Geometry: final body of the model. Coordinates: model frame, mm. Face numbers are marked on the shaded views. A direction names the side the tool comes from. Give positions to 0.01 mm unless a question says otherwise; leave off trailing zeros. Write each loop counter-clockwise with the first axis right and the second up, starting at its lowest first coordinate (ties: lowest second). Pieces come first, ordered by that corner, then holes. Notation, with made-up numbers: M 3,35.25 L 62,35.25 A26 cw 62,57.25 Z; hole C -10.5,-38.75 d8. An arc over 180 degrees is marked long. Use a Markdown table: item, result. Add a question column.
(1) Cut plane B-B (y = 0). Output: boundary loops of the cut face in (x, z).
(2) Draft query along Y for the marked faces 1, 2 and 3. Return one class per face: released by +Y, released by -Y, zero draft, split by the parting line, or undercut.
(3) Pin query (flat end, axial travel): pin 1 Ø3 at (x, z) = (-2.5, 8.5) entering from +Y; pin 2 Ø3 at (x, y) = (6.5, 0.5) entering from +Z; pin 3 Ø3 at (x, z) = (7, 2) entering from +Y. Return the tip coordinate at first contact, or that it passes through.
(4) Material intervals for L1, parallel to Z at x = -7.5, y = -0.25; L2, parallel to Y at x = -1, z = 4.25; L3, parallel to Y at x = 0.5, z = 8.75, sorted ascending.
(5) Reachability of the marked faces 4, 5, 6, 7 and 8 from +Z, -Z, +X, -X, +Y, -Y: full face, straight path, thin tool, end or side. Return the list, or none.
(6) Cut plane A-A (x = 0). Output: boundary loops of the cut face in (y, z).
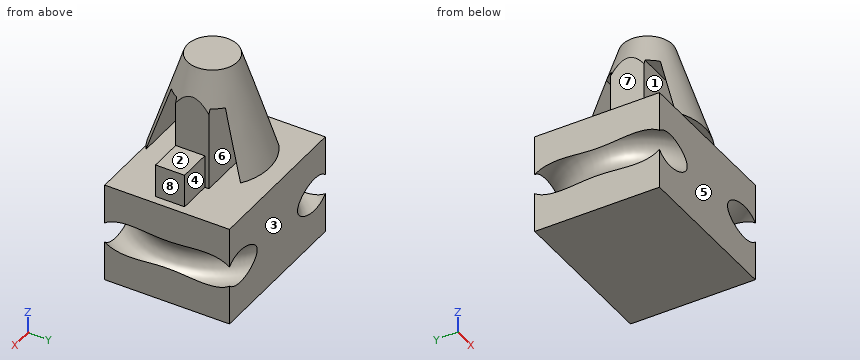
```python
from build123d import *

# Parameters (mm, degrees)
BOX008_W               = 10
BOX008_H               = 10
BOX008_DEPTH           = 5
BOX009_W               = 10
BOX009_H               = 10
BOX009_DEPTH           = 5
BOX006_W               = 10
BOX006_H               = 10
BOX006_DEPTH           = 15
BOX006_PLACEMENT_ANGLE = 90
BOX005_W               = 10
BOX005_H               = 10
BOX005_DEPTH           = 15
BOX002_W               = 20
BOX002_H               = 8
BOX002_DEPTH           = 18
BOX002_ROLL_ANGLE      = 16.999951
BOX003_W               = 20
BOX003_H               = 5
BOX003_DEPTH           = 10
CUT001_PLACEMENT_ANGLE = 180
BOX001_W               = 20
BOX001_H               = 8
BOX001_DEPTH           = 18
BOX001_ROLL_ANGLE      = 16.999951
BOX_W                  = 20
BOX_H                  = 5
BOX_DEPTH              = 10
TORUS_R                = 2
BOX007_W               = 19
BOX007_H               = 15
BOX007_DEPTH           = 12
BOX004_W               = 11
BOX004_H               = 3.5
BOX004_DEPTH           = 4


with BuildPart() as box008:
    # Box008 → Box008 (new body)
    with BuildSketch(Plane(origin=(-5, 5, -3), x_dir=(1, 0, 0), z_dir=(0, 0, 1))):
        with Locations((5, 5)):
            Rectangle(BOX008_W, BOX008_H)
    extrude(amount=BOX008_DEPTH)


with BuildPart() as box009:
    # Box009 → Box009 (new body)
    with BuildSketch(Plane(origin=(5, -4, -3), x_dir=(-1, 0, 0), z_dir=(0, 0, 1))):
        with Locations((5, 5)):
            Rectangle(BOX009_W, BOX009_H)
    extrude(amount=BOX009_DEPTH)


with BuildPart() as box006:
    # Box006 → Box006 (new body)
    with BuildSketch(Plane.XY):
        with Locations((5, 5)):
            Rectangle(BOX006_W, BOX006_H)
    extrude(amount=BOX006_DEPTH)


with BuildPart() as box006_1:
    # Box006 placement: moved
    add(box006.part.moved(Location((-4, -4, 0))).rotate(Axis((-4, -4, 0), (0, 0, 1)), BOX006_PLACEMENT_ANGLE))


with BuildPart() as box005:
    # Box005 → Box005 (new body)
    with BuildSketch(Plane(origin=(4, -4, 0), x_dir=(1, 0, 0), z_dir=(0, 0, 1))):
        with Locations((5, 5)):
            Rectangle(BOX005_W, BOX005_H)
    extrude(amount=BOX005_DEPTH)


with BuildPart() as box002:
    # Box002 → Box002 (new body)
    with BuildSketch(Plane.XY):
        with Locations((10, 4)):
            Rectangle(BOX002_W, BOX002_H)
    extrude(amount=BOX002_DEPTH)


with BuildPart() as box002_1:
    # Box002 roll: moved
    add(box002.part.rotate(Axis((0, 0, 0), (1, 0, 0)), BOX002_ROLL_ANGLE))


with BuildPart() as box002_2:
    # Box002 placement: moved
    add(box002_1.part.moved(Location((0, 17.17, -2.83))))


with BuildPart() as cu_a001:
    # Box003 → Box003 (new body)
    with BuildSketch(Plane(origin=(0, 12, 0), x_dir=(1, 0, 0), z_dir=(0, 0, 1))):
        with Locations((10, 2.5)):
            Rectangle(BOX003_W, BOX003_H)
    extrude(amount=BOX003_DEPTH)

    # Cut001: cut Box002
    add(box002_2.part, mode=Mode.SUBTRACT)


with BuildPart() as cu_a001_1:
    # Cut001 placement: moved
    add(cu_a001.part.moved(Location((10, 10, 0))).rotate(Axis((10, 10, 0), (0, 0, 1)), CUT001_PLACEMENT_ANGLE))


with BuildPart() as box001:
    # Box001 → Box001 (new body)
    with BuildSketch(Plane.XY):
        with Locations((10, 4)):
            Rectangle(BOX001_W, BOX001_H)
    extrude(amount=BOX001_DEPTH)


with BuildPart() as box001_1:
    # Box001 roll: moved
    add(box001.part.rotate(Axis((0, 0, 0), (1, 0, 0)), BOX001_ROLL_ANGLE))


with BuildPart() as box001_2:
    # Box001 placement: moved
    add(box001_1.part.moved(Location((0, 17.17, -2.83))))


with BuildPart() as cu_a:
    # Box → Box (new body)
    with BuildSketch(Plane(origin=(0, 12, 0), x_dir=(1, 0, 0), z_dir=(0, 0, 1))):
        with Locations((10, 2.5)):
            Rectangle(BOX_W, BOX_H)
    extrude(amount=BOX_DEPTH)

    # Cut: cut Box001
    add(box001_2.part, mode=Mode.SUBTRACT)


with BuildPart() as cu_a_1:
    # Cut placement: moved
    add(cu_a.part.moved(Location((-10, -10, 0))))


with BuildPart() as cut007:
    # Cone → Cone (revolve)
    with BuildSketch(Plane.XZ):
        Polygon((0, 0), (7.5, 0), (3, 14), (0, 14), align=None)
    revolve(axis=Axis((0, 0, 0), (0, 0, 1)))

    add(cu_a_1.part, mode=Mode.SUBTRACT)

    add(cu_a001_1.part, mode=Mode.SUBTRACT)

    # Cut004: cut Box005
    add(box005.part, mode=Mode.SUBTRACT)

    # Cut005: cut Box006
    add(box006_1.part, mode=Mode.SUBTRACT)

    # Cut006: cut Box009
    add(box009.part, mode=Mode.SUBTRACT)

    # Cut007: cut Box008
    add(box008.part, mode=Mode.SUBTRACT)


with BuildPart() as torus:
    # Torus → Torus (revolve)
    with BuildSketch(Plane(origin=(-0.5, 0, -6), x_dir=(1, 0, 0), z_dir=(0, -1, 0))):
        with Locations((10.5, 0)):
            Circle(TORUS_R)
    revolve(axis=Axis((-0.5, 0, -6), (0, 0, 1)))


with BuildPart() as cut008:
    # Box007 → Box007 (new body)
    with BuildSketch(Plane(origin=(-10, -7.5, -12), x_dir=(1, 0, 0), z_dir=(0, 0, 1))):
        with Locations((9.5, 7.5)):
            Rectangle(BOX007_W, BOX007_H)
    extrude(amount=BOX007_DEPTH)

    # Cut008: cut Torus
    add(torus.part, mode=Mode.SUBTRACT)


with BuildPart() as fusion:
    # Box004 → Box004 (new body)
    with BuildSketch(Plane(origin=(-3, -2, 0), x_dir=(1, 0, 0), z_dir=(0, 0, 1))):
        with Locations((5.5, 1.75)):
            Rectangle(BOX004_W, BOX004_H)
    extrude(amount=BOX004_DEPTH)

    # Fusion: union Cut007, Cut008
    add(cut007.part)
    add(cut008.part)


solid = fusion.part
```
Answer list:
| question | item | result |
|---|---|---|
| 1 | outline | M -10,-12 L 9,-12 L 9,-7.73 A2 cw 9,-4.27 L 9,0 L 8,0 L 8,4 L 4,4 L 4,10.89 L 3,14 L -3,14 L -4,10.89 L -4,0 L -10,0 L -10,-4.27 A2 cw -10,-7.73 Z |
| 2 | face 1 | undercut |
| 2 | face 2 | zero draft |
| 2 | face 3 | released by +Y |
| 3 | pin 1 | y = 4.9 |
| 3 | pin 2 | z = 4 |
| 3 | pin 3 | y = 1.5 |
| 4 | L1 | -12 to 0 |
| 4 | L2 | -6.05 to -5.01, -2 to 2, 5.01 to 6.05 |
| 4 | L3 | -4.66 to -3.63, -2 to 2, 3.63 to 4.66 |
| 5 | face 4 | +Z, +X, +Y |
| 5 | face 5 | +Z, -Z, +X, -X, -Y |
| 5 | face 6 | +X, -X |
| 5 | face 7 | +Z, -X, +Y, -Y |
| 5 | face 8 | +Z, +X, +Y, -Y |
| 6 | outline | M -7.5,-12 L 7.5,-12 L 7.5,0 L 2,0 L 2,10 L 3.25,10 L 5.69,2 L 6.86,2 L 3,14 L -3,14 L -6.86,2 L -5.69,2 L -3.25,10 L -2,10 L -2,0 L -7.5,0 Z |
